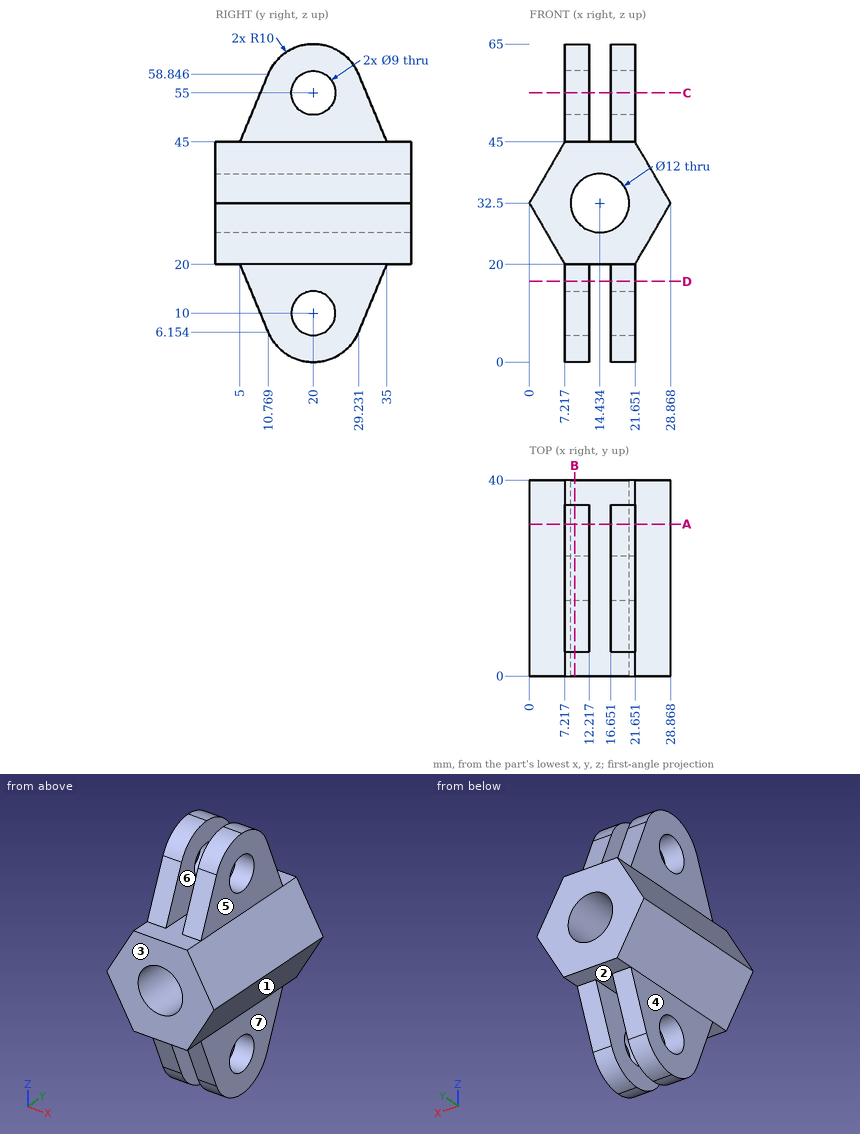
Geometry: see drawing. Coordinates: mm, zero at the bounding-box minimum. A direction names the side the tool comes from. Give positions to 0.01 mm unless a question says otherwise; leave off trailing zeros. Order: outer loops, then holes, each group sorted by start corner. A loop starts at its lowest first (then second) coordinate and runs counter-clockwise, first axis right, second up. Notation, with made-up numbers: (37, -26.5) -> (42, -26.5) arc R14 cw to (42, 0.5) -> close; hole circle Ø10 at (-40, 57). An arc over 180 degrees is marked (long way). Write each question's results on one line, items separated by ' | '. Start each with the question number.
1) Section A-A (y = 31). Return loops of the section in (x, z), then the cut area to 3 significant figures.
2) Section B-B (x = 9.25). Return loops of the section in (y, z), then the cut area to 3 significant figures.
3) Line query: line 1 (X direction, y = 24.5, z = 52); line 2 (Z direction, x = 9, y = 20) (1 decimal); line 3 (Z direction, x = 9.4, y = 20) (1 decimal). Output: solid intervals per line, ascending. Write a range as from..to.
4) Section C-C (z = 55). Return loops of the section in (x, y).
5) Set-up query: the marked faces 4, 5, 6 and 7. Return all of +Z, -Z, +X, -X, +Y, -Y with unobstructed straight access to the full face (end or side cutting, diameter ignored); none if empty.
6) First-contact query: pin 1 (6 mm diameter, centred on y = 23, z = 5, fed in from -X); pin 2 (6 mm diameter, centred on x = 21, y = 34.5, fed in from +Z); pin 3 (1.5 mm diameter, centred on y = 17.5, z = 41, fed in from +X); pin 4 (8 mm diameter, centred on y = 20, z = 10, fed in from -X). Flat tips, straight axial feed; report the tip coordinate or a pass-through.
7) Section D-D (z = 16.5). Return loops of the section in (x, y), then the cut area to 3 significant figures.
8) Draft query along X for the marked faces 1, 2 and 3. Return one class per face: pulls with the +X half, pulls with the -X half, needs draft (parallel to the pull), parting line crosses it, or undercut.
Calculated:
1) outline: (0, 32.5) -> (7.22, 20) -> (7.22, 10.4) -> (12.22, 10.4) -> (12.22, 20) -> (16.65, 20) -> (16.65, 10.4) -> (21.65, 10.4) -> (21.65, 20) -> (28.87, 32.5) -> (21.65, 45) -> (21.65, 54.6) -> (16.65, 54.6) -> (16.65, 45) -> (12.22, 45) -> (12.22, 54.6) -> (7.22, 54.6) -> (7.22, 45) -> close; hole circle Ø12 at (14.43, 32.5) | area: 620 mm2
2) outline: (0, 20) -> (5, 20) -> (10.77, 6.15) arc R10 ccw to (29.23, 6.15) -> (35, 20) -> (40, 20) -> (40, 29.48) -> (0, 29.48) -> close; (0, 35.52) -> (40, 35.52) -> (40, 45) -> (35, 45) -> (29.23, 58.85) arc R10 ccw to (10.77, 58.85) -> (5, 45) -> (0, 45) -> close; hole circle Ø9 at (20, 10); hole circle Ø9 at (20, 55) | area: 1,470 mm2
3) line 1: 7.22..12.22, 16.65..21.65 | line 2: 0..5.5, 14.5..30, 35..50.5, 59.5..65 | line 3: 0..5.5, 14.5..29.2, 35.8..50.5, 59.5..65
4) outline: (7.22, 9.17) -> (12.22, 9.17) -> (12.22, 15.5) -> (7.22, 15.5) -> close; (7.22, 24.5) -> (12.22, 24.5) -> (12.22, 30.83) -> (7.22, 30.83) -> close; (16.65, 9.17) -> (21.65, 9.17) -> (21.65, 15.5) -> (16.65, 15.5) -> close; (16.65, 24.5) -> (21.65, 24.5) -> (21.65, 30.83) -> (16.65, 30.83) -> close
5) face 4: -Z, -X, +Y, -Y | face 5: +Z, +X, +Y, -Y | face 6: +Z, +Y, -Y | face 7: -Z, +X, +Y, -Y
6) pin 1: x = 7.22 | pin 2: z = 53.4 | pin 3: x = 24.39 | pin 4: through
7) outline: (7.22, 6.46) -> (12.22, 6.46) -> (12.22, 33.54) -> (7.22, 33.54) -> close; (16.65, 6.46) -> (21.65, 6.46) -> (21.65, 33.54) -> (16.65, 33.54) -> close | area: 271 mm2
8) face 1: pulls with the +X half | face 2: undercut | face 3: needs draft
